Geometry check sheet. Reference: the model listing, model coordinates, mm. Round coordinates to 2 decimals unless told otherwise and drop trailing zeros. Order: outer loops, then holes, each group sorted by start corner. A loop starts at its lowest first (then second) coordinate and runs counter-clockwise, first axis right, second up.
(1) Sectioned sample at A-A (z = 435). Record the boundary of the cut face in (x, y), plus the area to 3 significant figures.
(2) Material ranges on line 1 along X through (y, z) = (1.85, 450); line 2 along Z through (x, y) = (-11, 1.8); line 3 along Y through (x, z) = (-10.5, 409), recorded low to high.
(3) Go/stop test with flat-tipped pins: pin 1 (2.5 mm diameter, centred on x = -12.5, z = 281, fed in from +Y); pin 2 (5 mm diameter, centred on y = 7.5, z = 299, fed in from +X); pin 3 (6 mm diameter, centred on x = 10.5, y = 22.5, fed in from +Z) (3 decimals); pin 4 (4 mm diameter, centred on y = 25, z = 441, fed in from -X). Record where each tip stops, or that it passes through.
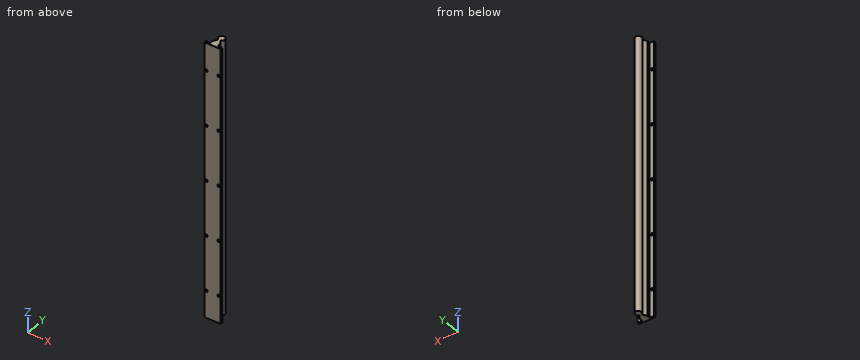
from build123d import *

# Parameters (mm, degrees)
BOSS_EXTRUDE1_DEPTH  = 500
SKETCH2_R            = 2.25
CUT_EXTRUDE1_DEPTH   = 502.06486606
LPATTERN1_COUNT      = 5
LPATTERN1_PITCH      = 100
LPATTERN1_COUNT_DIR2 = 2
LPATTERN1_PITCH_DIR2 = 22
FILLET1_R            = 0.5


with BuildPart() as part:
    # Sketch1 → Boss-Extrude1 (new body)
    with BuildSketch(Plane.XY):
        with BuildLine():
            Line((-15, 0), (15, 0))
            Line((15, 0), (15, 4))
            Line((15, 4), (7, 4))
            Line((7, 4), (7, 10))
            Line((7, 10), (2.259191805, 17.441578247))
            ThreePointArc((2.259191805, 17.441578247), (0, 29), (-2.259191805, 17.441578247))
            Line((-2.259191805, 17.441578247), (-7, 10))
            Line((-7, 10), (-7, 4))
            Line((-7, 4), (-15, 4))
            Line((-15, 4), (-15, 0))
        make_face()
    extrude(amount=BOSS_EXTRUDE1_DEPTH)

    # Sketch2 → Cut-Extrude1 (cut, through all)
    with BuildSketch(Plane.XZ):
        with Locations((-11, 50)):
            Circle(SKETCH2_R)
    cut_extrude1 = extrude(amount=-CUT_EXTRUDE1_DEPTH, mode=Mode.SUBTRACT)

    # LPattern1: Cut-Extrude1 5 × 2
    with Locations(*[(j * LPATTERN1_PITCH_DIR2, 0, i * LPATTERN1_PITCH) for i in range(LPATTERN1_COUNT) for j in range(LPATTERN1_COUNT_DIR2) if (i, j) != (0, 0)]):
        add(cut_extrude1, mode=Mode.SUBTRACT)

    # Fillet1
    fillet1_edges = [part.edges().sort_by_distance(p)[0] for p in [
        (-11, 4, 0),
        (-15, 2, 0),
        (0, 0, 0),
        (15, 2, 0),
        (11, 4, 0),
        (7, 7, 0),
        (4.629595903, 13.720789123, 0),
        (0, 29, 500),
        (0, 29, 0),
        (-4.629595903, 13.720789123, 0),
        (-7, 7, 0),
        (4.629595903, 13.720789123, 500),
        (7, 7, 500),
        (11, 4, 500),
        (15, 2, 500),
        (0, 0, 500),
        (-15, 2, 500),
        (-11, 4, 500),
        (-7, 7, 500),
        (-4.629595903, 13.720789123, 500),
    ]]
    fillet(fillet1_edges, radius=FILLET1_R)


solid = part.part
Answer below:
1. outline: (-15, 0) - (15, 0) - (15, 4) - (7, 4) - (7, 10) - (2.26, 17.44) arc R6 ccw (long way) to (-2.26, 17.44) - (-7, 10) - (-7, 4) - (-15, 4) - close
1. area: 385 mm2
2. line 1: x = -15 to -13.25, -8.75 to 8.75, 13.25 to 15
2. line 2: z = 0 to 47.75, 52.25 to 147.75, 152.25 to 247.75, 252.25 to 347.75, 352.25 to 447.75, 452.25 to 500
2. line 3: y = 0 to 4
3. pin 1: stops at y = 4
3. pin 2: stops at x = 7
3. pin 3: passes through
3. pin 4: stops at x = -6
